from build123d import *

# Parameters (mm, degrees)
F0_W     = 25
F0_H     = 24
F1_DEPTH = 0.5
F3_D     = 2.1
F4_W     = 20.8
F4_H     = 5.5
F5_DEPTH = 2.5
F6_W     = 8
F6_H     = 8
F7_DEPTH = 4.9


with BuildPart() as f1:
    # F0 (on Front) → F1 (new body, symmetric)
    with BuildSketch(Plane.XZ):
        Rectangle(F0_W, F0_H)
    extrude(amount=F1_DEPTH, both=True)

    # F3 (through all)
    with Locations(Plane.XZ.offset(0.5)):
        with Locations((-10.5, 2.5), (-10.5, -10), (10.5, 2.5), (10.5, -10)):
            Hole(F3_D / 2)

    # F4 (on face) → F5 (join)
    with BuildSketch(Plane(origin=(0, 0.5, 0), x_dir=(-1, 0, 0), z_dir=(0, 1, 0))):
        with Locations((0, 9.25)):
            Rectangle(F4_W, F4_H)
    extrude(amount=F5_DEPTH)

    # F6 (on face) → F7 (join)
    with BuildSketch(Plane.XZ.offset(0.5)):
        with Locations((0, 2.5)):
            Rectangle(F6_W, F6_H)
    extrude(amount=F7_DEPTH)


solid = f1.part
The model under review builds one solid part; all positions refer to its coordinate system, in mm. A direction names the side the tool comes from. Round coordinates to 2 decimals unless told otherwise and drop trailing zeros. Loops run counter-clockwise (first coordinate to the right, second up) from the corner with the lowest first, then second, coordinate; pieces in that order, holes last. Notation, with made-up numbers: (22.25, 86.5) -> (71.25, 86.5) arc R22 ccw to (71.25, 120.5) -> close; hole circle Ø10 at (16.5, 54.25). An arc over 180 degrees is marked (long way). One line per question, with ' | ' between items. Start each with the question number.
Item 1: Draft analysis for pull direction X (two halves, no side actions). For faces 1 (the face through (-12.5, 0, 0)), 2 (the face through (-11.5, 0.01, 2.82)), 3 (the face through (0, 3, 9)), 4 (the face through (-11.06, 0.01, -9.11)), state which applies: +X half, -X half, draft (parallel to the pull), parting line (faces both ways), or undercut.
Item 2: Machinability: for faces 5 (the face through (10.4, 2, 9)), 6 (the face through (0, -3, 6.5)), 7 (the face through (4, -3, 2)), 8 (the face through (0, 2, 6.5)), which of the approach directions +Z, -Z, +X, -X, +Y, -Y give a long, thin tool a straight path to every point of the face, cutting with its end or side? Answer none if there is none.
Item 3: Wall thickness on line 1 along Z through (x, y) = (-10.5, 0.3); line 2 along Y through (x, z) = (-3.5, 1); line 3 along Z through (x, y) = (1.25, -3): over which ranges is each line inside the solid? List them lowest first. Write a range as [from, to].
Item 4: Add section A-A, the plane z = -10. Write out the cut boundary in (x, y).
Item 5: Add section C-C, the plane x = 2. Write out the cut boundary in (y, z).
Item 6: Add section D-D, the plane z = 2.5. Write out the cut boundary in (x, y).
Item 7: For pin 1 (2.5 mm diameter, centred on x = 10.5, z = 2.5, fed in from +Y); pin 2 (1.7 mm diameter, centred on x = -10.5, z = 2.5, fed in from +Y); pin 3 (2.5 mm diameter, centred on y = -2, z = 2.5, fed in from +X); pin 4 (2.5 mm diameter, centred on x = 10.5, z = -10, fed in from -Y), all flat-tipped, find the tip position at first contact; note any pin that passes through.
Item 8: Add section B-B, the plane x = 9.75. Write out the cut boundary in (y, z), then the cut area to 3 significant figures.
Return value:
1) face 1: -X half | face 2: undercut | face 3: draft | face 4: undercut
2) face 5: +Z, -Z, +X, +Y | face 6: +Z, +X, -X, -Y | face 7: +Z, -Z, +X, -Y | face 8: -Z, +X, -X, +Y
3) line 1: z = [-12, -11.05], [-8.95, 1.45], [3.55, 12] | line 2: y = [-5.4, 0.5] | line 3: z = [-1.5, 6.5]
4) outline: (-12.5, -0.5) -> (-11.55, -0.5) -> (-11.55, 0.5) -> (-12.5, 0.5) -> close; (-9.45, -0.5) -> (9.45, -0.5) -> (9.45, 0.5) -> (-9.45, 0.5) -> close; (11.55, -0.5) -> (12.5, -0.5) -> (12.5, 0.5) -> (11.55, 0.5) -> close
5) outline: (-5.4, -1.5) -> (-0.5, -1.5) -> (-0.5, -12) -> (0.5, -12) -> (0.5, 6.5) -> (3, 6.5) -> (3, 12) -> (-0.5, 12) -> (-0.5, 6.5) -> (-5.4, 6.5) -> close
6) outline: (-12.5, -0.5) -> (-11.55, -0.5) -> (-11.55, 0.5) -> (-12.5, 0.5) -> close; (-9.45, -0.5) -> (-4, -0.5) -> (-4, -5.4) -> (4, -5.4) -> (4, -0.5) -> (9.45, -0.5) -> (9.45, 0.5) -> (-9.45, 0.5) -> close; (11.55, -0.5) -> (12.5, -0.5) -> (12.5, 0.5) -> (11.55, 0.5) -> close
7) pin 1: stops at y = 0.5 | pin 2: passes through | pin 3: stops at x = 4 | pin 4: stops at y = -0.5
8) outline: (-0.5, -12) -> (0.5, -12) -> (0.5, -10.73) -> (-0.5, -10.73) -> close; (-0.5, -9.27) -> (0.5, -9.27) -> (0.5, 1.77) -> (-0.5, 1.77) -> close; (-0.5, 3.23) -> (0.5, 3.23) -> (0.5, 6.5) -> (3, 6.5) -> (3, 12) -> (-0.5, 12) -> close | area: 34.8 mm2
